Model file for the job. Use its own axes, mm. Face numbers are marked on the shaded views. A direction names the side the tool comes from. Coordinates: 2 decimals unless noted, no trailing zeros. Order: outer loops, then holes, each group sorted by start corner. A loop starts at its lowest first (then second) coordinate and runs counter-clockwise, first axis right, second up. Notation, with made-up numbers: (66.5, 68.5) -> (75.5, 68.5) arc R35 cw to (75.5, 107.5) -> close; hole circle Ø5 at (-35.75, 52.5). An arc over 180 degrees is marked (long way). Return JSON: item names as keys, results as strings. Group by question number.
1) Flat gauge pins, fed straight in: pin 1 (1.5 mm diameter, centred on x = 26, z = -26, fed in from -Y); pin 2 (20.5 mm diameter, centred on x = 0, y = 0, fed in from -Z); pin 3 (1.5 mm diameter, centred on x = 12.5, z = -42, fed in from -Y). Where does each tip first touch, or does it go through?
2) Which spindle directions (+Z, -Z, +X, -X, +Y, -Y) get a long thin tool onto all of the face, cutting with end or side? Do the marked faces 1 and 2. Say none if no direction does.
3) Cut at A-A (x = 0). Write the cut outline in (y, z), and give its area (3 significant figures).
4) Probe line 1 (Y direction, x = 0, z = -56); line 2 (Y direction, x = 0, z = -40.5); line 3 (Z direction, x = -17.5, y = -29). List the from-to ranges inside material, lowest first.
5) Pull direction X, two halves, no side cores. Call the marked faces 3, 4, 5 and 6: +X half, -X half, draft (parallel to the pull), parting line (faces both ways), or undercut.
6) Cut at D-D (z = -55). Write the cut outline in (x, y).
7) Cut at C-C (z = -12). Write the cut outline in (x, y).
from build123d import *

# Parameters (mm, degrees)
CHAMFER1_SIZE   = 3.464101615
CHAMFER1_SIZE_2 = 6


with BuildPart() as part:
    # Sketch1 → Revolve1 (revolve)
    with BuildSketch(Plane(origin=(0, 0, 0), x_dir=(1, 0, 0), z_dir=(0, 1, 0)), mode=Mode.PRIVATE) as revolve1_sk:
        Polygon((0, 0), (0, 60.8), (-36, 60.8), (-36, 57.8), (-30, 57.8), (-30, 3), (-36, 3), (-36, 0), align=None)
    revolve(revolve1_sk.sketch.rotate(Axis((0, 0, 0), (0, 0, -1)), 180), axis=Axis((0, 0, 0), (0, 0, -1)))

    # Sketch7 → Cut-Revolve1 (revolve, cut)
    with BuildSketch(Plane(origin=(0, 0, 0), x_dir=(1, 0, 0), z_dir=(0, 1, 0))):
        Polygon((0, 60.8), (-11.1, 60.8), (-11.1, 53.5), (-9, 53.5), (-9, 7.3), (-11.1, 7.3), (-11.1, 0), (0, 0), align=None)
    revolve(axis=Axis((0, 0, -60.8), (0, 0, 1)), mode=Mode.SUBTRACT)

    # Chamfer1
    # the kernel refuses this chamfer: 6, 3.464101615 mm, written as the material it takes off along each edge
    with BuildSketch(Plane(origin=(0, 0, -57.8), x_dir=(1, 0, 0), z_dir=(0, 1, 0))) as chamfer1_piece_1_section:
        Polygon((36, CHAMFER1_SIZE), (36 - CHAMFER1_SIZE_2, 0), (36, 0), align=None)
    chamfer1_piece_1 = revolve(axis=Axis((0, 0, -57.8), (0, 0, -1)), mode=Mode.PRIVATE)
    chamfer1_piece_1 = chamfer1_piece_1 - Plane(origin=(0, 0, -57.8), x_dir=(1, 0, 0), z_dir=(0, 0, 1)) * Cylinder(30, 144, mode=Mode.PRIVATE)
    add(chamfer1_piece_1, mode=Mode.SUBTRACT)
    with BuildSketch(Plane(origin=(0, 0, -3), x_dir=(1, 0, 0), z_dir=(0, 1, 0))) as chamfer1_piece_2_section:
        Polygon((36 - CHAMFER1_SIZE_2, 0), (36, -CHAMFER1_SIZE), (36, 0), align=None)
    chamfer1_piece_2 = revolve(axis=Axis((0, 0, -3), (0, 0, -1)), mode=Mode.PRIVATE)
    chamfer1_piece_2 = chamfer1_piece_2 - Plane(origin=(0, 0, -3), x_dir=(1, 0, 0), z_dir=(0, 0, 1)) * Cylinder(30, 144, mode=Mode.PRIVATE)
    add(chamfer1_piece_2, mode=Mode.SUBTRACT)


solid = part.part
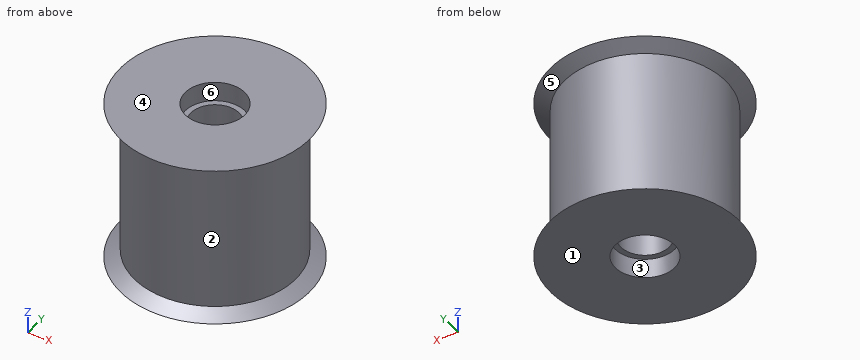
Answers below:
{
 "1": {"pin 1": "stops at y = -16.2", "pin 2": "stops at z = -53.5", "pin 3": "stops at y = -27.6"},
 "2": {"face 1": "-Z, +X, -X, +Y, -Y", "face 2": "none"},
 "3": {"outline": "(-35.2, -60.8) -> (-11.1, -60.8) -> (-11.1, -53.5) -> (-9, -53.5) -> (-9, -7.3) -> (-11.1, -7.3) -> (-11.1, 0) -> (-35.2, 0) -> (-30, -3) -> (-30, -57.8) -> close; (9, -53.5) -> (11.1, -53.5) -> (11.1, -60.8) -> (35.2, -60.8) -> (30, -57.8) -> (30, -3) -> (35.2, 0) -> (11.1, 0) -> (11.1, -7.3) -> (9, -7.3) -> close", "area": "2,520 mm^2"},
 "4": {"line 1": "y = -30 to -11.1, 11.1 to 30", "line 2": "y = -30 to -9, 9 to 30", "line 3": "z = -60.8 to -60.03, -0.77 to 0"},
 "5": {"face 3": "undercut", "face 4": "draft", "face 5": "parting line", "face 6": "undercut"},
 "6": {"outline": "circle Ø60 at (0, 0); hole circle Ø22.2 at (0, 0)"},
 "7": {"outline": "circle Ø60 at (0, 0); hole circle Ø18 at (0, 0)"}
}
